```python
from build123d import *

# Parameters (mm, degrees)
SKETCH1_R           = 1.2
SKETCH1_R_2         = 1.016
BOSS_EXTRUDE1_DEPTH = 1.778


with BuildPart() as part:
    # Sketch1 → Boss-Extrude1 (new body)
    with BuildSketch(Plane.XY):
        with BuildLine():
            ThreePointArc((-18.786436302, -4.117817235), (-20.050708925, -7.759998805), (-16.680479475, -9.632276912))
            ThreePointArc((-16.680479475, -9.632276912), (-4.834628254, -10.963744593), (4.131590393, -18.818928901))
            ThreePointArc((4.131590393, -18.818928901), (7.793176957, -20.037700838), (9.603735314, -16.629695609))
            ThreePointArc((9.603735314, -16.629695609), (10.808475978, -4.78617574), (18.757897672, 4.075373655))
            ThreePointArc((18.757897672, 4.075373655), (19.966132816, 7.95635676), (16.197476331, 9.479212735))
            ThreePointArc((16.197476331, 9.479212735), (4.341589411, 9.810476534), (-3.884701894, 18.354475699))
            ThreePointArc((-3.884701894, 18.354475699), (-7.540001964, 20.125778306), (-9.626354431, 16.640686499))
            ThreePointArc((-9.626354431, 16.640686499), (-10.896236616, 4.800764559), (-18.786436302, -4.117817235))
        make_face()
        with Locations((0, 8)):
            Circle(SKETCH1_R, mode=Mode.SUBTRACT)
        with Locations((-9.5, 0)):
            Circle(SKETCH1_R, mode=Mode.SUBTRACT)
        with Locations((9.5, 0)):
            Circle(SKETCH1_R, mode=Mode.SUBTRACT)
        with Locations((0, -8)):
            Circle(SKETCH1_R, mode=Mode.SUBTRACT)
        with Locations((17.255056752, 6.671807588)):
            Circle(SKETCH1_R_2, mode=Mode.SUBTRACT)
        with Locations((6.683111778, -17.263013667)):
            Circle(SKETCH1_R_2, mode=Mode.SUBTRACT)
        with Locations((-17.251709477, -6.691068694)):
            Circle(SKETCH1_R_2, mode=Mode.SUBTRACT)
        with Locations((-6.679764504, 17.243752562)):
            Circle(SKETCH1_R_2, mode=Mode.SUBTRACT)
    extrude(amount=BOSS_EXTRUDE1_DEPTH)


solid = part.part
```
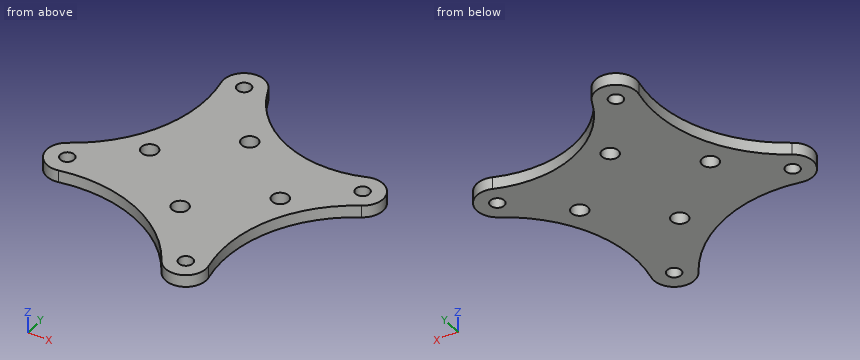
Work out the finished part from the listing and answer in its coordinate system (mm). Coordinates: 2 decimals unless noted, no trailing zeros. Loops run counter-clockwise (first coordinate to the right, second up) from the corner with the lowest first, then second, coordinate; pieces in that order, holes last.
1) Section D-D (y = 14) is taken. Give the vertices of the cut face in (x, z).
Results:
outline: (-9.27, 0) - (-1.27, 0) - (-1.27, 1.78) - (-9.27, 1.78) - close
2) Section C-C (z = 0.85) is taken. Give the number of separate pieces and of enclosed holes in the cut face, plus the area to 3 significant figures.
Results:
separate pieces: 1
enclosed holes: 8
area: 700 mm2
3) A flat-ended cylindrical pin translates along its axis: pin 1 (2 mm diameter, centred on x = 0, y = 8, fed in from -Z). Find the tip coordinate at first contact, or state that the pin passes through.
Results:
pin 1: passes through
4) Section A-A (x = 0) is taken. Give the vertices of the cut face in (y, z).
Results:
outline: (-13.99, 0) - (-9.2, 0) - (-9.2, 1.78) - (-13.99, 1.78) - close; (-6.8, 0) - (6.8, 0) - (6.8, 1.78) - (-6.8, 1.78) - close; (9.2, 0) - (12.67, 0) - (12.67, 1.78) - (9.2, 1.78) - close
5) Consider probe 1 along Y at (x, z) = (0, 0.25); probe 2 along X at (y, z) = (-1, 0.55); probe 3 along X at (y, z) = (-7, 0.7). Determine where each line is inside the solid, lowest interval first.
Results:
probe 1: y = -13.99 to -9.2, -6.8 to 6.8, 9.2 to 12.67
probe 2: x = -14.82 to -10.16, -8.84 to 8.84, 10.16 to 13.03
probe 3: x = -20.23 to -18.22, -16.28 to -0.66, 0.66 to 9.99
6) Section B-B (y = -0.5) is taken. Give the vertices of the cut face in (x, z), plus the area to 3 significant figures.
Results:
outline: (-14.35, 0) - (-10.59, 0) - (-10.59, 1.78) - (-14.35, 1.78) - close; (-8.41, 0) - (8.41, 0) - (8.41, 1.78) - (-8.41, 1.78) - close; (10.59, 0) - (13.42, 0) - (13.42, 1.78) - (10.59, 1.78) - close
area: 41.6 mm2
